Geometry: see drawing. Coordinates: mm, zero at the bounding-box minimum. A direction names the side the tool comes from. Give positions to 0.01 mm unless a question says otherwise; leave off trailing zeros. Loops run counter-clockwise (first coordinate to the right, second up) from the corner with the lowest first, then second, coordinate; pieces in that order, holes last. Notation, with made-up numbers: M -30,36 L -13,36 A23 cw -13,68 Z; hole C -33,-26 d7. An arc over 180 degrees is marked long. Answer in a Markdown table with one row per item.
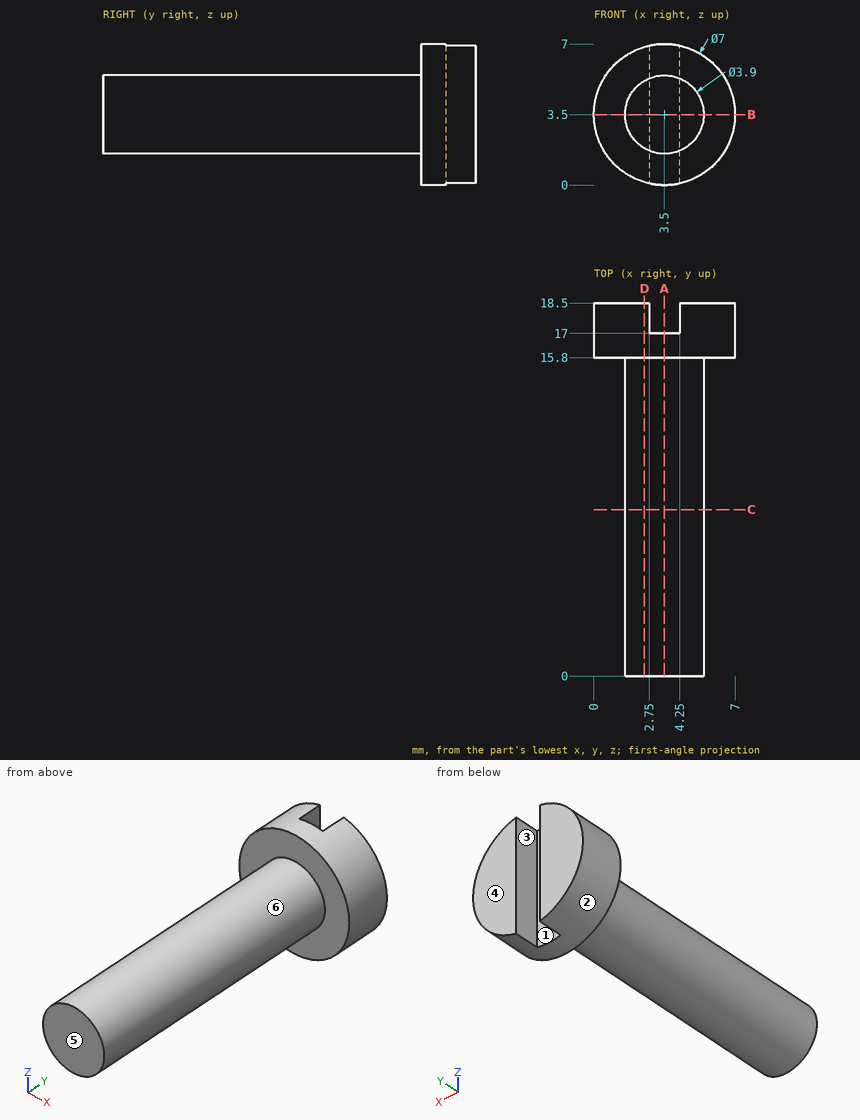
1) Pull-direction query (X, two-part tool) for the marked faces 1, 2, 3 and 4; classes: released by +X, released by -X, zero draft, split by the parting line, or undercut.
Reply:
| item | result |
|---|---|
| face 1 | undercut |
| face 2 | split by the parting line |
| face 3 | undercut |
| face 4 | zero draft |
2) Section C-C, the plane y = 8.25. Return loops of the section in (x, z), then the cut area to 3 significant figures.
Reply:
| item | result |
|---|---|
| outline | C 3.5,3.5 d3.9 |
| area | 11.9 mm² |
3) Section B-B, the plane z = 3.5. Return loops of the section in (x, y).
Reply:
| item | result |
|---|---|
| outline | M 0,15.8 L 1.55,15.8 L 1.55,0 L 5.45,0 L 5.45,15.8 L 7,15.8 L 7,18.5 L 4.25,18.5 L 4.25,17 L 2.75,17 L 2.75,18.5 L 0,18.5 Z |
4) Set-up query: the marked faces 5 and 6. Return all of +Z, -Z, +X, -X, +Y, -Y with unobstructed straight access to the full face (end or side cutting, diameter ignored); none if empty.
Reply:
| item | result |
|---|---|
| face 5 | +Z, -Z, +X, -X, -Y |
| face 6 | -Y |
5) Section A-A, the plane x = 3.5. Return loops of the section in (y, z).
Reply:
| item | result |
|---|---|
| outline | M 0,1.55 L 15.8,1.55 L 15.8,0 L 17,0 L 17,7 L 15.8,7 L 15.8,5.45 L 0,5.45 Z |
6) Section D-D, the plane x = 2.5. Return loops of the section in (y, z), then the cut area to 3 significant figures.
Reply:
| item | result |
|---|---|
| outline | M 0,1.83 L 15.8,1.83 L 15.8,0.15 L 18.5,0.15 L 18.5,6.85 L 15.8,6.85 L 15.8,5.17 L 0,5.17 Z |
| area | 71.0 mm² |
7) Material intervals for L1, parallel to Y at x = 0.75, z = 5.5; L2, parallel to Y at x = 3.5, z = 3.75; L3, parallel to Z at x = 3.25, y = 5.75, sorted ascending.
Reply:
| item | result |
|---|---|
| L1 | y = 15.8 to 18.5 |
| L2 | y = 0 to 17 |
| L3 | z = 1.57 to 5.43 |
8) Pin query (flat end, axial travel): pin 1 Ø3 at (x, y) = (4, 10.5) entering from -Z; pin 2 Ø1 at (y, z) = (15.5, 5.5) entering from +X; pin 3 Ø3 at (x, y) = (4.5, 9) entering from +Z; pin 4 Ø0.8 at (y, z) = (17.5, 3) entering from +X. Return the tip coordinate at first contact, or that it passes through.
Reply:
| item | result |
|---|---|
| pin 1 | stops at z = 1.55 |
| pin 2 | stops at x = 6.61 |
| pin 3 | stops at z = 5.45 |
| pin 4 | stops at x = 7 |
